from build123d import *

# Parameters (mm, degrees)
F0_W     = 79.375
F0_H     = 79.375
F1_DEPTH = 165.1
F2_W     = 76.2
F2_H     = 76.2
F3_DEPTH = 162.56
F4_R     = 1.27
F6_DEPTH = 79.376


with BuildPart() as f1:
    # F0 (on Top) → F1 (new body)
    with BuildSketch(Plane.XY):
        Rectangle(F0_W, F0_H)
    extrude(amount=F1_DEPTH)

    # F2 (on face) → F3 (cut)
    with BuildSketch(Plane(origin=(0, 0, 0), x_dir=(1, 0, 0), z_dir=(0, 0, -1))):
        Rectangle(F2_W, F2_H)
    extrude(amount=-F3_DEPTH, mode=Mode.SUBTRACT)

    # F4
    f4_edges = [f1.edges().sort_by_distance(p)[0] for p in [
        (39.6875, -39.6875, 82.55),
        (39.6875, 0, 165.1),
        (39.6875, 39.6875, 82.55),
        (-39.6875, -39.6875, 82.55),
        (0, -39.6875, 165.1),
        (0, 39.6875, 165.1),
        (-39.6875, 39.6875, 82.55),
        (-39.6875, 0, 165.1),
    ]]
    fillet(f4_edges, radius=F4_R)

    # F5 (on face) → F6 (cut, through all)
    with BuildSketch(Plane.YZ.offset(39.6875)):
        Polygon((46.8884, 13.7033), (-38.4175, 0), (46.8884, -9.378617), align=None)
    extrude(amount=-F6_DEPTH, mode=Mode.SUBTRACT)


solid = f1.part
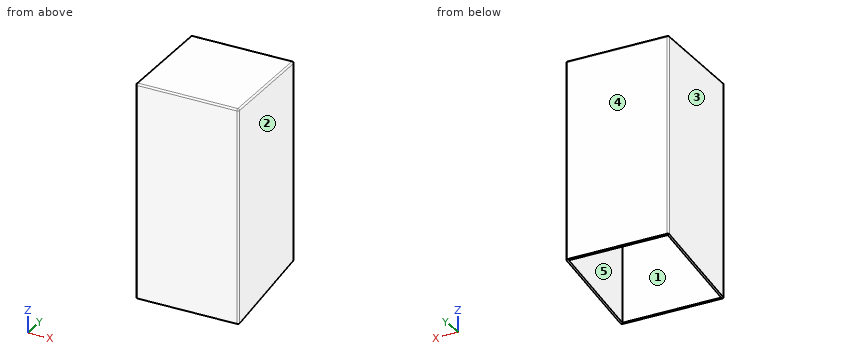
Input: part model. Units: mm. Frame: model coordinates. Face numbers are marked on the shaded views. A direction names the side the tool comes from. Give positions to 0.01 mm unless a question says otherwise; leave off trailing zeros. Order: outer loops, then holes, each group sorted by start corner. A loop starts at its lowest first (then second) coordinate and runs counter-clockwise, first axis right, second up.
Q1. Draft query along Y for the marked faces 3, 4 and 5. Return one class per face: +Y half, -Y half, draft (parallel to the pull), parting line (faces both ways), or undercut.
Checked values:
face 3: draft
face 4: +Y half
face 5: undercut
Q2. Section B-B on x = 23. Output: boundary loops of the cut face in (y, z), and give its area (3 significant figures).
Checked values:
outline: (-39.69, 0) - (-38.42, 0) - (-38.1, 0.05) - (-38.1, 162.56) - (38.1, 162.56) - (38.1, 12.29) - (39.69, 12.55) - (39.69, 163.83) arc R1.27 ccw to (38.42, 165.1) - (-38.42, 165.1) arc R1.27 ccw to (-39.69, 163.83) - close
area: 697 mm2
Q3. Contact query for a flat-ended pin moving along its axis: pin 1 Ø1 at (x, y) = (-8, -28.5) entering from -Z. Output: stop coordinate, or through.
Checked values:
pin 1: stops at z = 162.56
Q4. Section C-C on y = -33.5. Output: boundary loops of the cut face in (x, z), and give its area (3 significant figures).
Checked values:
outline: (-39.69, 0.79) - (-38.1, 0.79) - (-38.1, 162.56) - (38.1, 162.56) - (38.1, 0.79) - (39.69, 0.79) - (39.69, 163.83) arc R1.27 ccw to (38.42, 165.1) - (-38.42, 165.1) arc R1.27 ccw to (-39.69, 163.83) - close
area: 715 mm2
Q5. Section D-D on z = 10.5. Output: boundary loops of the cut face in (x, y).
Checked values:
outline: (-39.69, -38.42) arc R1.27 ccw to (-38.42, -39.69) - (38.42, -39.69) arc R1.27 ccw to (39.69, -38.42) - (39.69, 26.95) - (38.1, 26.95) - (38.1, -38.1) - (-38.1, -38.1) - (-38.1, 26.95) - (-39.69, 26.95) - close
Q6. Ray query, probe 1 along Y at (x, z) = (-28.5, 59); probe 2 along Z at (x, y) = (-21.5, 35). Return the intervals inside material, ascending.
Checked values:
probe 1: y = -39.69 to -38.1, 38.1 to 39.69
probe 2: z = 162.56 to 165.1
Q7. Set-up query: the marked faces 1 and 2. Return all of +Z, -Z, +X, -X, +Y, -Y with unobstructed straight access to the full face (end or side cutting, diameter ignored); none if empty.
Checked values:
face 1: -Z
face 2: +Z, -Z, +X, +Y, -Y
Q8. Section A-A on z = 54.5. Output: boundary loops of the cut face in (x, y).
Checked values:
outline: (-39.69, -38.42) arc R1.27 ccw to (-38.42, -39.69) - (38.42, -39.69) arc R1.27 ccw to (39.69, -38.42) - (39.69, 38.42) arc R1.27 ccw to (38.42, 39.69) - (-38.42, 39.69) arc R1.27 ccw to (-39.69, 38.42) - close; hole (-38.1, -38.1) - (38.1, -38.1) - (38.1, 38.1) - (-38.1, 38.1) - close
